Check sheet for the modelled part. Datum: model origin and axes. Units: mm. Face numbers are marked on the shaded views. Round coordinates to 2 decimals unless told otherwise and drop trailing zeros. Loops run counter-clockwise (first coordinate to the right, second up) from the corner with the lowest first, then second, coordinate; pieces in that order, holes last. Notation, with made-up numbers: (80, 43.25) -> (102, 43.25) arc R22 cw to (102, 79.25) -> close; hole circle Ø8 at (-4.75, 52.25). An arc over 180 degrees is marked (long way). Return JSON: item names as keys, results as strings.
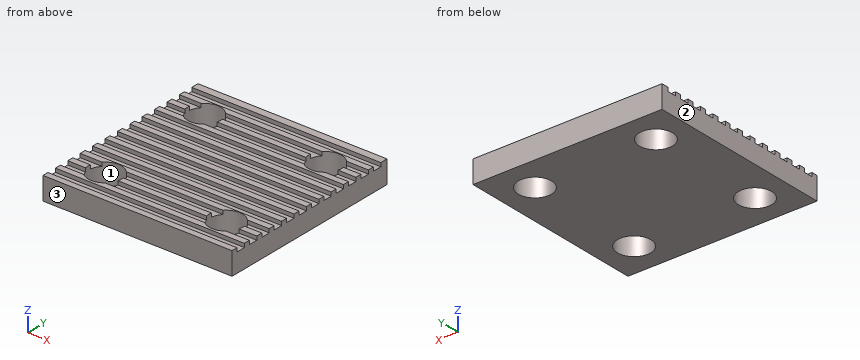
from build123d import *

# Parameters (mm, degrees)
F0_W     = 25
F0_H     = 25
F1_DEPTH = 3
F2_D     = 4.4
F3_W     = 1.2
F3_H     = 0.5
F4_DEPTH = 25.001


with BuildPart() as f1:
    # F0 (on Top) → F1 (new body)
    with BuildSketch(Plane.XY):
        Rectangle(F0_W, F0_H)
    extrude(amount=F1_DEPTH)

    # F2 (through all)
    with Locations(Plane(origin=(0, 0, 0), x_dir=(1, 0, 0), z_dir=(0, 0, -1))):
        with Locations((-8, -8), (8, -8), (8, 8), (-8, 8)):
            Hole(F2_D / 2)

    # F3 (on face) → F4 (cut, through all)
    with BuildSketch(Plane.YZ.offset(12.5)):
        with Locations((-11.1, 2.75)):
            Rectangle(F3_W, F3_H)
        with Locations((-9.1, 2.75)):
            Rectangle(F3_W, F3_H)
        with Locations((-7.1, 2.75)):
            Rectangle(F3_W, F3_H)
        with Locations((-5.1, 2.75)):
            Rectangle(F3_W, F3_H)
        with Locations((-3.1, 2.75)):
            Rectangle(F3_W, F3_H)
        with Locations((-1.1, 2.75)):
            Rectangle(F3_W, F3_H)
        with Locations((0.9, 2.75)):
            Rectangle(F3_W, F3_H)
        with Locations((2.9, 2.75)):
            Rectangle(F3_W, F3_H)
        with Locations((4.9, 2.75)):
            Rectangle(F3_W, F3_H)
        with Locations((6.9, 2.75)):
            Rectangle(F3_W, F3_H)
        with Locations((8.9, 2.75)):
            Rectangle(F3_W, F3_H)
        with Locations((10.9, 2.75)):
            Rectangle(F3_W, F3_H)
    extrude(amount=-F4_DEPTH, mode=Mode.SUBTRACT)


solid = f1.part
Q1. Section check B-B (z = 1.6). Record the boundary of the cut face in (x, y).
Results list:
{"outline": "(-12.5, -12.5) -> (12.5, -12.5) -> (12.5, 12.5) -> (-12.5, 12.5) -> close; hole circle Ø4.4 at (-8, -8); hole circle Ø4.4 at (-8, 8); hole circle Ø4.4 at (8, -8); hole circle Ø4.4 at (8, 8)"}
Q2. Go/stop test with flat-tipped pins: pin 1 (3.5 mm diameter, centred on x = -8, y = 8, fed in from +Z); pin 2 (0.6 mm diameter, centred on x = -11, y = 7, fed in from +Z). Record where each tip stops, or that it passes through.
Results list:
{"pin 1": "through", "pin 2": "z = 2.5"}
Q3. Draft check along X on the marked faces 1, 2 and 3. Enter one of: released by +X, released by -X, zero draft, split by the parting line, or undercut.
Results list:
{"face 1": "undercut", "face 2": "released by -X", "face 3": "zero draft"}
Q4. Section check A-A (y = 8). Record the boundary of the cut face in (x, z), then the cut area to 3 significant figures.
Results list:
{"outline": "(-12.5, 0) -> (-10.2, 0) -> (-10.2, 3) -> (-12.5, 3) -> close; (-5.8, 0) -> (5.8, 0) -> (5.8, 3) -> (-5.8, 3) -> close; (10.2, 0) -> (12.5, 0) -> (12.5, 3) -> (10.2, 3) -> close", "area": "48.6 mm^2"}
Q5. Section check C-C (x = -8). Count the separate pieces of the cut face and the enclosed holes in it, then the cut area to 3 significant figures.
Results list:
{"separate pieces": "3", "enclosed holes": "0", "area": "43.8 mm^2"}
Q6. Material ranges on line 1 (X direction, y = 8, z = 1.25); line 2 (X direction, y = -9.5, z = 2.35), recorded low to high.
Results list:
{"line 1": "-12.5 to -10.2, -5.8 to 5.8, 10.2 to 12.5", "line 2": "-12.5 to -9.61, -6.39 to 6.39, 9.61 to 12.5"}
